Autodesk Inventor part; units mm, degrees
ref_plane "YZ Plane" through (0, 0, 0) normal (1, 0, 0) x (0, 1, 0)
ref_plane "XZ Plane" through (0, 0, 0) normal (0, 1, 0) x (-1, 0, 0)
ref_plane "XY Plane" through (0, 0, 0) normal (0, 0, 1) x (1, 0, 0)
sketch "Sketch1" plane through (0, 0, 0) normal (1, 0, 0) x (0, 1, 0)
  line L0 (14.6318, 23.7403) -> (-20.3682, 23.7403)
  line L1 (-20.3682, 23.7403) -> (-20.3682, -26.2597)
  line L2 (-20.3682, -26.2597) -> (-5.3682, -26.2597)
  line L3 (14.6318, -1.2597) -> (14.6318, 23.7403)
  line L4 (14.6318, -1.2597) -> (-5.3682, -1.2597)
  line L5 (-5.3682, -1.2597) -> (-5.3682, -26.2597)
  point P0 (0, 0)
  dimension "d8" = 35
  dimension "d9" = 25
  dimension "d10" = 20
  dimension "d11" = 25
  dimension "d12" = 50
extrude "Extrusion1" add sketch "Sketch1" along normal blind 20
fillet "Fillet1" radius 10 2 edges at (20, 14.6318, 11.2403) (0, 14.6318, 11.2403)
sketch "Sketch3" plane through (0, -20.3682, 23.7403) normal (0, 0, 1) x (1, 0, 0)
  circle A0 centre (10, 25) radius 1.5
  arc A1 (20, 25) -> (0, 25) centre (10, 25) ccw
  point P0 (0, 20.3682)
  dimension "d5" = 3
extrude "Extrusion2" add sketch "Sketch3" along normal blind 20
properties part number "Motor"
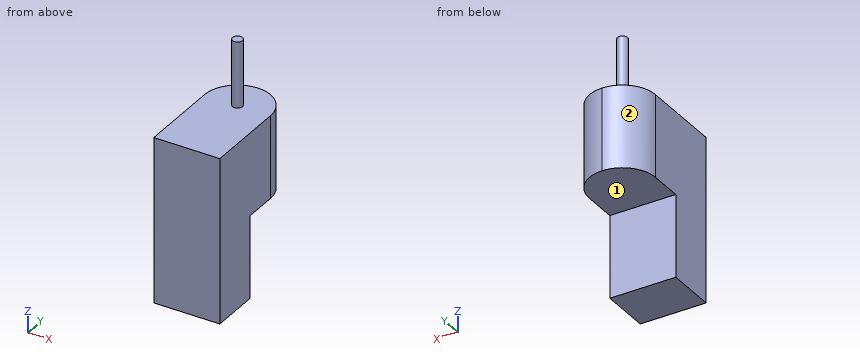
Input: part model. Units: mm. Frame: model coordinates. Face numbers are marked on the shaded views. A direction names the side the tool comes from. Coordinates: 2 decimals unless noted, no trailing zeros. Write each loop counter-clockwise with the first axis right and the second up, starting at its lowest first coordinate (ties: lowest second). Pieces come first, ordered by that corner, then holes.
1) Section C-C on x = 14.5. Output: boundary loops of the cut face in (y, z), and give its area (3 significant figures).
2) Pin query (flat end, axial travel): pin 1 Ø10 at (x, z) = (13, -13.5) entering from +Y; pin 2 Ø2 at (x, y) = (10, -8) entering from +Z; pin 3 Ø1 at (x, y) = (5, 3) entering from -Z. Return the tip coordinate at first contact, or that it passes through.
3) Material intervals for line 1 along Z through (x, y) = (11, 5.5); line 2 along Z through (x, y) = (11.25, 10); line 3 along Y through (x, z) = (9.75, -0.5), sorted ascending.
4) Section D-D on z = 25.5. Output: boundary loops of the cut face in (x, y), and give its area (3 significant figures).
5) Set-up query: the marked faces 1 and 2. Return all of +Z, -Z, +X, -X, +Y, -Y with unobstructed straight access to the full face (end or side cutting, diameter ignored); none if empty.
6) Section B-B on y = -4. Output: boundary loops of the cut face in (x, z).
7) Section A-A on z = -22. Output: boundary loops of the cut face in (x, y).
Check result:
1. outline: (-20.37, -26.26) - (-5.37, -26.26) - (-5.37, -1.26) - (13.56, -1.26) - (13.56, 23.74) - (-20.37, 23.74) - close
1. area: 1,220 mm2
2. pin 1: stops at y = -5.37
2. pin 2: stops at z = 23.74
2. pin 3: stops at z = -1.26
3. line 1: z = -1.26 to 43.74
3. line 2: z = -1.26 to 23.74
3. line 3: y = -20.37 to 14.63
4. outline: circle Ø3 at (10, 4.63)
4. area: 7.07 mm2
5. face 1: -Z, +X, -X, +Y
5. face 2: +Z, -Z, -X, +Y
6. outline: (0, -1.26) - (20, -1.26) - (20, 23.74) - (0, 23.74) - close
7. outline: (0, -20.37) - (20, -20.37) - (20, -5.37) - (0, -5.37) - close
